Autodesk Inventor part; units mm, degrees
ref_plane "YZ Plane" through (0, 0, 0) normal (1, 0, 0) x (0, 1, 0)
ref_plane "XZ Plane" through (0, 0, 0) normal (0, 1, 0) x (-1, 0, 0)
ref_plane "XY Plane" through (0, 0, 0) normal (0, 0, 1) x (1, 0, 0)
sketch "Sketch1" plane through (0, 0, 0) normal (1, 0, 0) x (0, 1, 0)
  line L0 (0, 0) -> (30.75, 0)
  line L1 (30.75, 0) -> (30.75, -30.75)
  line L2 (30.75, -30.75) -> (0, -30.75)
  line L3 (0, -30.75) -> (0, 0)
  line L4 (32.75, -32.75) -> (32.75, 2)
  line L5 (32.75, 2) -> (-2, 2)
  line L6 (-2, 2) -> (-2, -32.75)
  line L7 (-2, -32.75) -> (32.75, -32.75)
  circle A0 centre (30.75, 0) radius 1.25
  circle A1 centre (30.75, -30.75) radius 1.25
  circle A2 centre (0, -30.75) radius 1.25
  circle A3 centre (0, 0) radius 1.25
  line L8 (-4, 4) -> (34.75, 4)
  line L9 (34.75, 4) -> (34.75, -34.75)
  line L10 (34.75, -34.75) -> (-4, -34.75)
  line L11 (-4, -34.75) -> (-4, 4)
  circle A4 centre (7.375, -7.375) radius 1.25
  circle A5 centre (7.375, -23.375) radius 1.25
  circle A6 centre (23.375, -23.375) radius 1.25
  circle A7 centre (23.375, -7.375) radius 1.25
  dimension "d0" = 30.75
  dimension "d1" = 30.75
  dimension "d2" = 2
  dimension "d3" = 2.5
  dimension "d4" = 2
  dimension "d14" = 2.5
extrude "Extrusion3" add sketch "Sketch1" along normal blind 1 contours L0 A0 L1 A1 L2 A2 L3 A3 | L7 L6 L5 L4 | L8 L9 L10 L11
sketch "Sketch3" plane through (1, 0, 0) normal (1, 0, 0) x (0, 0, -1)
  line L0 (-4, -4) -> (34.75, -4)
  line L1 (34.75, -4) -> (34.75, 34.75)
  line L2 (-4, -4) -> (34.75, -4)
  line L3 (34.75, -4) -> (34.75, 34.75)
  line L4 (34.75, 34.75) -> (-4, 34.75)
  line L5 (-4, 34.75) -> (-4, -4)
  line L6 (-2, -2) -> (32.75, -2)
  line L7 (32.75, -2) -> (32.75, 32.75)
  line L8 (32.75, 32.75) -> (-2, 32.75)
  line L9 (-2, 32.75) -> (-2, -2)
  point P0 (0, 0)
  dimension "d17" = 2
extrude "Extrusion4" add sketch "Sketch3" along normal blind 1
sketch "Sketch4" plane through (2, 0, 0) normal (1, 0, 0) x (0, 0, -1)
  line L0 (-2, 32.75) -> (-2, -2)
  line L1 (-2, 15.375) -> (-2, 23.375)
  line L2 (-2, 23.375) -> (-4, 23.375)
  line L3 (-4, 34.75) -> (-4, -4)
  line L4 (-4, 23.375) -> (-4, 7.375)
  line L5 (-4, 7.375) -> (-2, 7.375)
  line L6 (-2, 7.375) -> (-2, 15.375)
  point P0 (0, 0)
  dimension "d20" = 8
  dimension "d21" = 16
extrude "Extrusion5" cut sketch "Sketch4" against normal blind 1
properties part number "Mag_Shield_Back"
The model under review builds one solid part; all positions refer to its coordinate system, in mm. A direction names the side the tool comes from. Round coordinates to 2 decimals unless told otherwise and drop trailing zeros. Loops run counter-clockwise (first coordinate to the right, second up) from the corner with the lowest first, then second, coordinate; pieces in that order, holes last. Notation, with made-up numbers: (-23.5, 3.5) - (-10.5, 3.5) arc R9 ccw to (-10.5, 15.5) - close; hole circle Ø11 at (50.25, 49.25). An arc over 180 degrees is marked (long way). Use a Markdown table: item, result. Add a question column.
Q1. Machinability: for faces 1 (the face through (1.5, 23.375, 3)), 2 (the face through (0.493, 31.905, -30.271)), 3 (the face through (1.5, -2, -15.1)), which of the approach directions +Z, -Z, +X, -X, +Y, -Y give a long, thin tool a straight path to every point of the face, cutting with its end or side? Answer none if there is none.
Q2. Add section B-B (z = -30.75). State the section outline as (x, y) points, plus the area to 4 significant figures.
Q3. For probe 1 along Y at (x, z) = (0.45, 0); probe 2 along Y at (x, z) = (1.25, -16); probe 3 along Z at (x, y) = (0.55, 6.5), list the stretches that pass through material, from the lowest coordinate up.
Q4. The part is to be moulded in two halves that separate along Y. For faces 4 (the face through (0.49, -0.27, -29.53)), 5 (the face through (1, -4, -15)), 6 (the face through (1, 15, -34.75)), say which applies: pulls with the +Y half, pulls with the -Y half, needs draft (parallel to the pull), parting line crosses it, or undercut.
Q5. Add section D-D (y = 4). State the section outline as (x, z) points, plus the area to 4 significant figures.
Q6. Insertion check: pin 1 Ø17.5 at (y, z) = (12.5, -20.5) entering from +X; pin 2 Ø3 at (y, z) = (0, 0) entering from -X; pin 3 Ø0.5 at (x, y) = (1.5, 17) entering from +Z. Each pin has a flat end and moves straight along its axis. Give the tip position at first contact, or say it passes through.
Q7. Add section C-C (x = 0.3). State how many separate pieces and enclosed holes the cut face has, plus the area to 3 significant figures.
Q8. Add section A-A (y = 30.75). State the section outline as (x, z) points.
Worked answers:
| question | item | result |
|---|---|---|
| 1 | face 1 | +Z, +X |
| 1 | face 2 | +X, -X |
| 1 | face 3 | +X |
| 2 | outline | (0, -4) - (2, -4) - (2, -2) - (1, -2) - (1, -1.25) - (0, -1.25) - close; (0, 1.25) - (1, 1.25) - (1, 29.5) - (0, 29.5) - close; (0, 32) - (1, 32) - (1, 32.75) - (2, 32.75) - (2, 34.75) - (0, 34.75) - close |
| 2 | area | 37.75 mm² |
| 3 | probe 1 | -4 to -1.25, 1.25 to 29.5, 32 to 34.75 |
| 3 | probe 2 | -4 to -2, 32.75 to 34.75 |
| 3 | probe 3 | -34.75 to -24.27, -22.48 to -8.27, -6.48 to 4 |
| 4 | face 4 | undercut |
| 4 | face 5 | pulls with the -Y half |
| 4 | face 6 | needs draft |
| 5 | outline | (0, -34.75) - (2, -34.75) - (2, -32.75) - (1, -32.75) - (1, 2) - (2, 2) - (2, 4) - (0, 4) - close |
| 5 | area | 42.75 mm² |
| 6 | pin 1 | x = 1 |
| 6 | pin 2 | x = 0 |
| 6 | pin 3 | z = -32.75 |
| 7 | separate pieces | 1 |
| 7 | enclosed holes | 8 |
| 7 | area | 1,460 mm² |
| 8 | outline | (0, -34.75) - (2, -34.75) - (2, -32.75) - (1, -32.75) - (1, -32) - (0, -32) - close; (0, -29.5) - (1, -29.5) - (1, -1.25) - (0, -1.25) - close; (0, 1.25) - (1, 1.25) - (1, 2) - (2, 2) - (2, 4) - (0, 4) - close |
